Geometry: final body of the model. Coordinates: model frame, mm. A direction names the side the tool comes from. Give positions to 0.01 mm unless a question says otherwise; leave off trailing zeros. Write each loop counter-clockwise with the first axis right and the second up, starting at its lowest first coordinate (ties: lowest second). Pieces come first, ordered by that corner, then holes. Notation, with made-up numbers: (-21.5, 31.25) - (0.5, 31.25) arc R19 cw to (0.5, 47.25) - close; hole circle Ø10 at (3.25, 78.5). An arc over 180 degrees is marked (long way). One line per question, with ' | ' between items. Start each with the question number.
```python
from build123d import *

# Parameters (mm, degrees)
CROQUIS2_W              = 6
CROQUIS2_H              = 6
SALIENTE_EXTRUIR2_DEPTH = 2


# Read off the part's stored shape, not the designer's step: Saliente-Extruir1
with BuildPart() as part:
    # Saliente-Extruir1 outline → Saliente-Extruir1 (revolve)
    with BuildSketch(Plane.XY):
        Polygon((0, 10), (0, -2), (2, 0), (2, 10), align=None)
    revolve(axis=Axis((0, 0, 0), (0, 1, 0)))

    # Croquis2 → Saliente-Extruir2 (add)
    with BuildSketch(Plane(origin=(0, 10, 0), x_dir=(1, 0, 0), z_dir=(0, 1, 0))):
        Rectangle(CROQUIS2_W, CROQUIS2_H)
    extrude(amount=SALIENTE_EXTRUIR2_DEPTH)


solid = part.part
```
1) Reachability of faces 1 (the flat face through (0, 12, 0)), 2 (the flat face through (-1, 10, -2)) from +Z, -Z, +X, -X, +Y, -Y: full face, straight path, thin tool, end or side. Return the list, or none.
2) First-contact query: pin 1 Ø1.5 at (y, z) = (2.5, -1) entering from -X; pin 2 Ø1 at (y, z) = (0.5, 1) entering from -X; pin 3 Ø1.5 at (x, z) = (-0.5, -1.5) entering from -Y. Flat tips, straight axial feed; report the tip coordinate or a pass-through.
3) Line query: L1, parallel to Y at x = -1.9, z = 2.1; L2, parallel to Y at x = -0.7, z = -1; L3, parallel to Z at x = -0.85, y = -1. Output: solid intervals per line, ascending.
4) Section A-A, the plane z = 2.2. Output: boundary loops of the cut face in (x, y).
5) Section B-B, the plane y = 2.5. Output: boundary loops of the cut face in (x, z), plus the area to 3 significant figures.
Answer key:
1) face 1: +Z, -Z, +X, -X, +Y | face 2: -Y
2) pin 1: x = -1.98 | pin 2: x = -1.94 | pin 3: y = -1.17
3) L1: 10 to 12 | L2: -0.78 to 12 | L3: -0.53 to 0.53
4) outline: (-3, 10) - (3, 10) - (3, 12) - (-3, 12) - close
5) outline: circle Ø4 at (0, 0) | area: 12.6 mm^2
